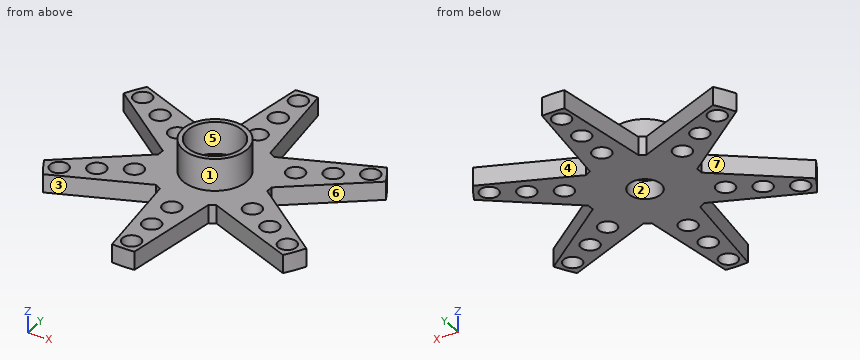
```python
from build123d import *

# Parameters (mm, degrees)
SKETCH1_R           = 1
BOSS_EXTRUDE3_DEPTH = 2
SKETCH2_R           = 1.75
CUT_EXTRUDE2_DEPTH  = 2
SKETCH3_R           = 3.5
SKETCH3_R_2         = 3
BOSS_EXTRUDE4_DEPTH = 3.5


with BuildPart() as part:
    # Sketch1 → Boss-Extrude3 (new body)
    with BuildSketch(Plane.XY):
        with BuildLine():
            ThreePointArc((1.229444159, 15.952694665), (0, 16), (-1.229444159, 15.952694665))
            Line((-1.229444159, 15.952694665), (-2.666890983, 5.374727201))
            ThreePointArc((-2.666890983, 5.374727201), (-3, 5.196152423), (-3.321204803, 4.996958941))
            Line((-3.321204803, 4.996958941), (-13.200716759, 9.041077207))
            ThreePointArc((-13.200716759, 9.041077207), (-13.856406461, 8), (-14.430160918, 6.911617458))
            Line((-14.430160918, 6.911617458), (-5.988095786, 0.37776826))
            ThreePointArc((-5.988095786, 0.37776826), (-5.999999995, -0.000251411), (-5.988064107, -0.378270083))
            Line((-5.988064107, -0.378270083), (-14.426795427, -6.918639585))
            ThreePointArc((-14.426795427, -6.918639585), (-13.85251149, -8.006742498), (-13.196315379, -9.04750023))
            Line((-13.196315379, -9.04750023), (-3.320786342, -4.997237044))
            ThreePointArc((-3.320786342, -4.997237044), (-2.999782432, -5.196278029), (-2.666890983, -5.374727201))
            Line((-2.666890983, -5.374727201), (-1.229444159, -15.952694665))
            ThreePointArc((-1.229444159, -15.952694665), (0, -16), (1.229444159, -15.952694665))
            Line((1.229444159, -15.952694665), (2.666890983, -5.374727201))
            ThreePointArc((2.666890983, -5.374727201), (3, -5.196152423), (3.321204803, -4.996958941))
            Line((3.321204803, -4.996958941), (13.200716759, -9.041077207))
            ThreePointArc((13.200716759, -9.041077207), (13.856406461, -8), (14.430160918, -6.911617458))
            Line((14.430160918, -6.911617458), (5.988095786, -0.37776826))
            ThreePointArc((5.988095786, -0.37776826), (5.999999995, 0.000251411), (5.988064107, 0.378270083))
            Line((5.988064107, 0.378270083), (14.426795427, 6.918639585))
            ThreePointArc((14.426795427, 6.918639585), (13.85251149, 8.006742498), (13.196315379, 9.04750023))
            Line((13.196315379, 9.04750023), (3.320786342, 4.997237044))
            ThreePointArc((3.320786342, 4.997237044), (2.999782432, 5.196278029), (2.666890983, 5.374727201))
            Line((2.666890983, 5.374727201), (1.229444159, 15.952694665))
        make_face()
        with Locations((0, 7.5)):
            Circle(SKETCH1_R, mode=Mode.SUBTRACT)
        with Locations((0, 11)):
            Circle(SKETCH1_R, mode=Mode.SUBTRACT)
        with Locations((0, 14.5)):
            Circle(SKETCH1_R, mode=Mode.SUBTRACT)
        with Locations((-6.495190528, 3.75)):
            Circle(SKETCH1_R, mode=Mode.SUBTRACT)
        with Locations((-12.557368355, 7.25)):
            Circle(SKETCH1_R, mode=Mode.SUBTRACT)
        with Locations((-9.526279442, 5.5)):
            Circle(SKETCH1_R, mode=Mode.SUBTRACT)
        with Locations((12.557368355, 7.25)):
            Circle(SKETCH1_R, mode=Mode.SUBTRACT)
        with Locations((6.495190528, 3.75)):
            Circle(SKETCH1_R, mode=Mode.SUBTRACT)
        with Locations((9.526279442, 5.5)):
            Circle(SKETCH1_R, mode=Mode.SUBTRACT)
        with Locations((-6.495190528, -3.75)):
            Circle(SKETCH1_R, mode=Mode.SUBTRACT)
        with Locations((-12.557368355, -7.25)):
            Circle(SKETCH1_R, mode=Mode.SUBTRACT)
        with Locations((-9.526279442, -5.5)):
            Circle(SKETCH1_R, mode=Mode.SUBTRACT)
        with Locations((12.557368355, -7.25)):
            Circle(SKETCH1_R, mode=Mode.SUBTRACT)
        with Locations((6.495190528, -3.75)):
            Circle(SKETCH1_R, mode=Mode.SUBTRACT)
        with Locations((9.526279442, -5.5)):
            Circle(SKETCH1_R, mode=Mode.SUBTRACT)
        with Locations((0, -7.5)):
            Circle(SKETCH1_R, mode=Mode.SUBTRACT)
        with Locations((0, -14.5)):
            Circle(SKETCH1_R, mode=Mode.SUBTRACT)
        with Locations((0, -11)):
            Circle(SKETCH1_R, mode=Mode.SUBTRACT)
    extrude(amount=BOSS_EXTRUDE3_DEPTH)

    # Sketch2 → Cut-Extrude2 (cut)
    with BuildSketch(Plane.XY.offset(2)):
        Circle(SKETCH2_R)
    extrude(amount=-CUT_EXTRUDE2_DEPTH, mode=Mode.SUBTRACT)

    # Sketch3 → Boss-Extrude4 (add)
    with BuildSketch(Plane.XY.offset(2)):
        Circle(SKETCH3_R)
        Circle(SKETCH3_R_2, mode=Mode.SUBTRACT)
    extrude(amount=BOSS_EXTRUDE4_DEPTH)


solid = part.part
```
Read the model definition and answer for the solid it produces. Units are mm, in the model's axes. Face numbers are marked on the shaded views. A direction names the side the tool comes from. Coordinates: 2 decimals unless noted, no trailing zeros. Loops run counter-clockwise (first coordinate to the right, second up) from the corner with the lowest first, then second, coordinate; pieces in that order, holes last.
(1) The part is cut by section C-C (z = 3.3). Determine the outline of the cut face in (x, y), and give its area (3 significant figures).
Solution:
outline: circle Ø7 at (0, 0); hole circle Ø6 at (0, 0)
area: 10.2 mm2
(2) A tool of negligible diameter and unlimited length cuts with its end or side. For the marked faces 1, 2, 3 and 4, from which of +Z, -Z, +X, -X, +Y, -Y can it reach the whole face along a straight path? Write none if from no direction.
Solution:
face 1: +Z
face 2: +Z, -Z
face 3: +Z, -Z, -Y
face 4: +Z, -Z, +Y
(3) The part is cut by section D-D (y = 11). Determine the outline of the cut face in (x, z).
Solution:
outline: (-1.9, 0) - (-1, 0) - (-1, 2) - (-1.9, 2) - close; (1, 0) - (1.9, 0) - (1.9, 2) - (1, 2) - close
(4) The mould has two halves that part along X. Classify the marked faces 5, 6 and 7: released by +X, released by -X, zero draft, split by the parting line, or undercut.
Solution:
face 5: undercut
face 6: released by +X
face 7: released by -X
(5) Consider line 1 along X through (y, z) = (-3.5, 0.9); line 2 along Y through (x, z) = (2, 3.1); line 3 along Z through (x, y) = (-1.25, 7). Determine where each line is inside the solid, lowest interval first.
Solution:
line 1: x = -10.02 to -7.46, -5.53 to 5.53, 7.46 to 10.02
line 2: y = -2.87 to -2.24, 2.24 to 2.87
line 3: z = 0 to 2
(6) The part is cut by section A-A (y = 0). Determine the outline of the cut face in (x, z).
Solution:
outline: (-6, 0) - (-1.75, 0) - (-1.75, 2) - (-3, 2) - (-3, 5.5) - (-3.5, 5.5) - (-3.5, 2) - (-6, 2) - close; (1.75, 0) - (6, 0) - (6, 2) - (3.5, 2) - (3.5, 5.5) - (3, 5.5) - (3, 2) - (1.75, 2) - close
(7) The part is cut by section B-B (x = 12.25). Determine the outline of the cut face in (y, z).
Solution:
outline: (-8.65, 0) - (-8.2, 0) - (-8.2, 2) - (-8.65, 2) - close; (-6.3, 0) - (-5.22, 0) - (-5.22, 2) - (-6.3, 2) - close; (5.23, 0) - (6.3, 0) - (6.3, 2) - (5.23, 2) - close; (8.2, 0) - (8.66, 0) - (8.66, 2) - (8.2, 2) - close
(8) Flat-ended cylindrical pins translate along their axes: pin 1 Ø3 at (x, y) = (0, 7.5) entering from +Z; pin 2 Ø1.8 at (x, y) = (-12.56, -7.25) entering from -Z; pin 3 Ø3 at (x, z) = (-2, 2) entering from +Y; pin 4 Ø1 at (y, z) = (11, 1) entering from +X. Find the tip coordinate at first contact, or state that the pin passes through.
Solution:
pin 1: stops at z = 2
pin 2: passes through
pin 3: stops at y = 15.99
pin 4: stops at x = 1.97
